Here's how the part is built. I have some questions about the finished solid (model axes, mm). A direction names the side the tool comes from. Coordinates: 2 decimals unless noted, no trailing zeros. Write each loop counter-clockwise with the first axis right and the second up, starting at its lowest first coordinate (ties: lowest second). Pieces come first, ordered by that corner, then holes. Notation, with made-up numbers: M -8.75,74 L 37.25,74 A26 ccw 37.25,94 Z; hole C 60,55.25 d9. An arc over 180 degrees is marked long. Use a Markdown table: item, result.
Autodesk Inventor part; units mm, degrees
ref_plane "YZ Plane" through (0, 0, 0) normal (1, 0, 0) x (0, 1, 0)
ref_plane "XZ Plane" through (0, 0, 0) normal (0, 1, 0) x (-1, 0, 0)
ref_plane "XY Plane" through (0, 0, 0) normal (0, 0, 1) x (1, 0, 0)
sketch "Sketch1" plane through (0, 0, 0) normal (0, 1, 0) x (-1, 0, 0)
  line L0 (-72.2313, -152.4) -> (72.2313, -152.4)
  line L1 (72.2313, -152.4) -> (72.2312, 152.4)
  line L2 (72.2312, 152.4) -> (-72.2312, 152.4)
  line L3 (-72.2312, 152.4) -> (-72.2313, -152.4)
  line L4 (-72.2313, -152.4) -> (72.2312, 152.4) construction
  line L5 (72.2313, -152.4) -> (-72.2312, 152.4) construction
  point P0 (0, 0)
  dimension "d0" = 144.4625
  dimension "d1" = 304.8
extrude "Extrusion1" add sketch "Sketch1" against normal blind 19.05
sketch "Sketch2" plane through (0, 0, 0) normal (0, 1, 0) x (1, 0, 0)
  line L0 (72.2312, -152.4) -> (-72.2312, -152.4)
  line L1 (-57.2312, -152.4) -> (57.2312, -152.4)
  line L2 (57.2312, -152.4) -> (57.2312, -182.4)
  line L3 (57.2312, -182.4) -> (-57.2312, -182.4)
  line L4 (-57.2312, -182.4) -> (-57.2312, -152.4)
  line L5 (-72.2313, 152.4) -> (-72.2312, -152.4)
  line L6 (72.2312, -152.4) -> (72.2313, 152.4)
  point P0 (0, 0)
  dimension "d4" = 15
  dimension "d5" = 15
  dimension "d6" = 30
extrude "Extrusion2" add sketch "Sketch2" against normal blind 19.05
sketch "Sketch3" plane through (0, 0, 0) normal (0, 1, 0) x (1, 0, 0)
  line L0 (-49.2312, -174.4) -> (49.2312, -174.4)
  line L1 (49.2312, -174.4) -> (49.2312, -154.4)
  line L2 (49.2312, -154.4) -> (-49.2312, -154.4)
  line L3 (-49.2312, -154.4) -> (-49.2312, -174.4)
  line L4 (-57.2312, -152.4) -> (-57.2312, -182.4)
  line L5 (-57.2312, -182.4) -> (57.2312, -182.4)
  line L6 (-72.2312, -152.4) -> (-57.2312, -152.4)
  line L7 (57.2312, -182.4) -> (57.2312, -152.4)
  point P0 (0, 0)
  point P1 (-57.2312, -167.4)
  dimension "d9" = 8
  dimension "d10" = 8
  dimension "d11" = 2
  dimension "d12" = 8
extrude "Extrusion3" cut sketch "Sketch3" against normal blind 19.05
fillet "Fillet1" radius 10 1 edges at (57.2312, -9.525, 182.4)
fillet "Fillet2" radius 10 1 edges at (-57.2312, -9.525, 182.4)
fillet "Fillet3" radius 10 1 edges at (-49.2312, -9.525, 174.4)
fillet "Fillet4" radius 10 1 edges at (49.2312, -9.525, 174.4)
properties material "Wood (Maple)"
1. Suppose I cut it at B-B on z = 158.5. Write out the boundary of the cut face in (x, y).
Answers follow:
| item | result |
|---|---|
| outline | M -57.23,-19.05 L -49.23,-19.05 L -49.23,0 L -57.23,0 Z; M 49.23,-19.05 L 57.23,-19.05 L 57.23,0 L 49.23,0 Z |
2. Suppose I cut it at C-C on y = -16. Write out the boundary of the cut face in (x, z), and give its area (3 significant figures).
Answers follow:
| item | result |
|---|---|
| outline | M -72.23,-152.4 L 72.23,-152.4 L 72.23,152.4 L 57.23,152.4 L 57.23,172.4 A10 ccw 47.23,182.4 L -47.23,182.4 A10 ccw -57.23,172.4 L -57.23,152.4 L -72.23,152.4 Z; hole M -49.23,154.4 L 49.23,154.4 L 49.23,164.4 A10 ccw 39.23,174.4 L -39.23,174.4 A10 ccw -49.23,164.4 Z |
| area | 45,500 mm2 |
3. Will these pins go through, and if not, where does the flat tip stop? pin 1 Ø8 at (y, z) = (-10.5, 161) entering from +X; pin 2 Ø9.5 at (y, z) = (-13.5, 165) entering from -X.
Answers follow:
| item | result |
|---|---|
| pin 1 | stops at x = 57.23 |
| pin 2 | stops at x = -57.23 |
4. We'd pull the mould along X, two halves only. Please class faces 5 (the face through (1, -9, 154.4)), 6 (the face through (65, -9, 152.4)), 7 (the face through (-54.22, -9.66, 179.55)): +X half, -X half, draft (parallel to the pull), parting line (faces both ways), or undercut.
Answers follow:
| item | result |
|---|---|
| face 5 | undercut |
| face 6 | draft |
| face 7 | -X half |
5. Which directions (+Z, -Z, +X, -X, +Y, -Y) give clear straight access to the entire face, cutting with the end or side of a thin tool? Please do faces 1 (the face through (57.231, -9, 162)), 2 (the face through (49.231, -9, 159)), 3 (the face through (1, 0, 17)), 4 (the face through (-57.231, -9, 163)).
Answers follow:
| item | result |
|---|---|
| face 1 | +Z, +X, +Y, -Y |
| face 2 | +Y, -Y |
| face 3 | +Z, -Z, +X, -X, +Y |
| face 4 | +Z, -X, +Y, -Y |
6. Suppose I cut it at A-A on x = 0.5. Write out the boundary of the cut face in (y, z), and give its area (3 significant figures).
Answers follow:
| item | result |
|---|---|
| outline | M -19.05,-152.4 L 0,-152.4 L 0,154.4 L -19.05,154.4 Z; M -19.05,174.4 L 0,174.4 L 0,182.4 L -19.05,182.4 Z |
| area | 6,000 mm2 |
7. I need wall thicknesses on probe 1 along Z at (x, y) = (-16.5, -1.75); probe 2 along Z at (x, y) = (-66, -6.75); probe 3 along Z at (x, y) = (-46, -8). Which ranges of each line are inside material? Lowest first, please.
Answers follow:
| item | result |
|---|---|
| probe 1 | z = -152.4 to 154.4, 174.4 to 182.4 |
| probe 2 | z = -152.4 to 152.4 |
| probe 3 | z = -152.4 to 154.4, 171.76 to 182.4 |
